Model file for the job. Use its own axes, mm. A direction names the side the tool comes from. Give positions to 0.01 mm unless a question says otherwise; leave off trailing zeros. Order: outer loops, then holes, each group sorted by start corner. A loop starts at its lowest first (then second) coordinate and runs counter-clockwise, first axis right, second up. Notation, with made-up numbers: (24, 54.5) -> (47, 54.5) arc R14 cw to (47, 62.5) -> close; hole circle Ø7 at (23.5, 68.25). An arc over 180 degrees is marked (long way). Use CSV: the item, a comma, the result in double quotes. Start each with the question number.
1. Cut at D-D on z = 16. List the corners of the cut face in (x, y), then the cut area to 3 significant figures.
2. Pull direction Z, two halves, no side cores. Call faces 4 (the flat face through (3, -1, 31)), 5 (the flat face through (-1, 3, 0)), 6 (the cylindrical face through (4.25, -0.163, 28.412)): released by +Z, released by -Z, zero draft, split by the parting line, or undercut.
3. Cut at A-A on y = 0. Give the number of separate pieces and of enclosed holes in the cut face, then the cut area to 3 significant figures.
4. 3-axis set-ups, long thin cutter, end or side, ignore diameter. For faces 1 (the cylindrical face through (2.769, -5.323, 26.814)), 2 (the conical face through (0.553, -4.213, 8.608)), 3 (the cylindrical face through (0.163, 4.25, 28.412)): which of +Z, -Z, +X, -X, +Y, -Y reach the whole face in a straight line?
5. Wall check: line 1 (Y direction, x = 0, z = 22.5); line 2 (Y direction, x = 0.25, z = 4); line 3 (X direction, y = -1, z = 11). Give the ranges that are in metal, low to high. Write a range as from..to.
6. Drop flat-ended pins along their axis: pin 1 (4 mm diameter, centred on x = 0.5, z = 9.5, fed in from +Y); pin 2 (1 mm diameter, centred on x = 0.5, y = 3, fed in from -Z); pin 3 (5 mm diameter, centred on x = -3.5, z = 16, fed in from -Y); pin 4 (6 mm diameter, centred on x = -3.5, z = 15, fed in from -Y). Give the stop position or say it passes through.
7. Cut at C-C on z = 2. List the corners of the cut face in (x, y), then the cut area to 3 significant figures.
```python
from build123d import *

# Parameters (mm, degrees)
SKETCH1_R               = 4.5
SKETCH1_R_2             = 2.75
BOSS_EXTRUDE1_DEPTH     = 21
DRAFT1_ANGLE            = -1.16
SKETCH2_R               = 6
SKETCH2_R_2             = 2.75
BOSS_EXTRUDE2_DEPTH     = 10
FILLET2_R               = 5
CUT_EXTRUDE1_REACH      = 35.779
CUT_EXTRUDE1_END_RADIUS = 2.75
SKETCH4_R               = 1.25
CIRPATTERN1_COUNT       = 2
CIRPATTERN1_ANGLE       = 90


with BuildPart() as part:
    # Sketch1 → Boss-Extrude1 (new body)
    with BuildSketch(Plane.XY):
        with Locations(Location((0, 0, 0), (0, 0, 180))):
            Circle(SKETCH1_R)
        with Locations(Location((0, 0, 0), (0, 0, 180))):
            Circle(SKETCH1_R_2, mode=Mode.SUBTRACT)
    extrude(amount=BOSS_EXTRUDE1_DEPTH)

    # Draft1
    draft1_faces = [part.faces().sort_by_distance(p)[0] for p in [
        (4.5, 0, 10.5),
    ]]
    draft(draft1_faces, Plane.XY.offset(21), DRAFT1_ANGLE)

    # Sketch2 → Boss-Extrude2 (add)
    with BuildSketch(Plane.XY.offset(21)):
        Circle(SKETCH2_R)
        with Locations(Location((0, 0, 0), (0, 0, 180))):
            Circle(SKETCH2_R_2, mode=Mode.SUBTRACT)
    extrude(amount=BOSS_EXTRUDE2_DEPTH)

    # Fillet1: read off the stored shape, not the designer's step
    # Fillet1 outline → Fillet1 (revolve)
    with BuildSketch(Plane.XZ):
        with BuildLine():
            Line((6, 21), (4.42833376, 21))
            Line((4.42833376, 21), (4.42833376, 17.460679283))
            ThreePointArc((4.42833376, 17.460679283), (4.857597383, 19.388677437), (6, 21))
        make_face()
    revolve(axis=Axis((0, 0, 0), (0, 0, 1)))

    # Fillet2
    fillet2_edges = [part.edges().sort_by_distance(p)[0] for p in [
        (-6, 0, 21),
    ]]
    fillet(fillet2_edges, radius=FILLET2_R)

    # Cut-Extrude1: up to this cylinder (the profile starts outside it)
    cut_extrude1_end = Plane(origin=(0, 0, 27.172961), z_dir=(0, 0, -1)) * Cylinder(CUT_EXTRUDE1_END_RADIUS, 78.058, mode=Mode.PRIVATE)
    # Sketch4 → Cut-Extrude1 (cut, up to the surface)
    with BuildSketch(Plane(origin=(6, 0, 31), x_dir=(0, 0, -1), z_dir=(1, 0, 0)), mode=Mode.PRIVATE) as cut_extrude1_sk1:
        with Locations(Location((3.827038513, 0, 0), (0, 0, 90))):
            Circle(SKETCH4_R)
    cut_extrude1_tool1 = extrude(cut_extrude1_sk1.sketch, amount=-CUT_EXTRUDE1_REACH, mode=Mode.PRIVATE) - cut_extrude1_end
    cut_extrude1 = cut_extrude1_tool1.solids().sort_by_distance((6, 0, 27.172961))[0]
    add(cut_extrude1, mode=Mode.SUBTRACT)

    # CirPattern1: Cut-Extrude1 ×2 about axis
    cirpattern1_axis = Axis((0, 0, 0), (0, 0, 1))
    for i in range(1, CIRPATTERN1_COUNT):
        add(cut_extrude1.rotate(cirpattern1_axis, i * CIRPATTERN1_ANGLE / (CIRPATTERN1_COUNT - 1)), mode=Mode.SUBTRACT)


solid = part.part
```
Verdict:
1,outline,"circle Ø8.8 at (0, 0); hole circle Ø5.5 at (0, 0)"
1,area,"37.0 mm^2"
2,face 4,"released by +Z"
2,face 5,"released by -Z"
2,face 6,"undercut"
3,separate pieces,"3"
3,enclosed holes,"0"
3,area,"124 mm^2"
4,face 1,"+Z, -Z"
4,face 2,"-Z"
4,face 3,"+Y"
5,line 1,"-5.99..-2.75, 2.75..5.99"
5,line 2,"-4.15..-2.74, 2.74..4.15"
5,line 3,"-4.18..-2.56, 2.56..4.18"
6,pin 1,"y = 4.31"
6,pin 2,"z = 0"
6,pin 3,"y = -4.29"
6,pin 4,"y = -4.36"
7,outline,"circle Ø8.23 at (0, 0); hole circle Ø5.5 at (0, 0)"
7,area,"29.4 mm^2"
